Read the model definition and answer for the solid it produces. Units are mm, in the model's axes. A direction names the side the tool comes from. Give positions to 0.01 mm unless a question says otherwise; leave off trailing zeros. Loops run counter-clockwise (first coordinate to the right, second up) from the corner with the lowest first, then second, coordinate; pieces in that order, holes last. Notation, with made-up numbers: (81, -33.75) -> (92, -33.75) arc R20 cw to (92, -10.75) -> close; hole circle Ø4 at (17, 36). An arc over 180 degrees is marked (long way). Return JSON: item names as keys, results as strings. Group by question number.
Autodesk Inventor part; units mm, degrees
ref_plane "YZ Plane" through (0, 0, 0) normal (1, 0, 0) x (0, 1, 0)
ref_plane "XZ Plane" through (0, 0, 0) normal (0, 1, 0) x (-1, 0, 0)
ref_plane "XY Plane" through (0, 0, 0) normal (0, 0, 1) x (1, 0, 0)
sketch "草图2" plane through (0, 0, 0) normal (1, 0, 0) x (0, 1, 0)
  arc A0 (-53.1995, 32.7287) -> (-53.1995, 62.7287) centre (4.8952, 47.7287) ccw
  line L0 (4.8952, 17.7287) -> (24.8952, 17.7287)
  line L1 (24.8952, 17.7287) -> (24.8952, 77.7287)
  line L2 (24.8952, 77.7287) -> (-15.1048, 77.7287)
  line L3 (-15.1048, 77.7287) -> (-15.1048, 17.7287)
  line L4 (-15.1048, 17.7287) -> (4.8952, 17.7287)
  arc A1 (-53.1995, 62.7287) -> (-53.1995, 32.7287) centre (4.8952, 47.7287) ccw
  point P0 (0, 0)
extrude "拉伸2" add sketch "草图2" along normal blind 4
sketch "草图3" plane through (4, 4.8952, 47.7287) normal (1, 0, 0) x (0, 0, -1)
  line L0 (-9, 58) -> (9, 58)
  line L1 (9, 58) -> (9, 54)
  line L2 (9, 54) -> (-9, 54)
  line L3 (-9, 54) -> (-9, 58)
  line L4 (0, -74) -> (0, 175)
  line L5 (0, 0) -> (111.1859, 0)
  line L6 (-9, -58) -> (9, -58)
  line L7 (9, -58) -> (9, -54)
  line L8 (9, -54) -> (-9, -54)
  line L9 (-9, -54) -> (-9, -58)
  line L10 (54, 9) -> (58, 9)
  line L11 (58, 9) -> (58, -9)
  line L12 (58, -9) -> (54, -9)
  line L13 (54, -9) -> (54, 9)
  line L14 (-54, 9) -> (-58, 9)
  line L15 (-58, 9) -> (-58, -9)
  line L16 (-58, -9) -> (-54, -9)
  line L17 (-54, -9) -> (-54, 9)
  dimension "d21" = 18
  dimension "d22" = 4
  dimension "d23" = 18
  dimension "d24" = 4
  dimension "d25" = 108
  dimension "d26" = 108
extrude "拉伸3" add sketch "草图3" along normal blind 18
sketch "草图4" plane through (4, -4.1048, -10.2713) normal (0, 0, -1) x (-1, 0, 0)
  line L0 (-4.5, 27) -> (-4.5, -16)
  line L1 (0, 69) -> (0, -51)
  line L2 (0, 0) -> (-18, 0)
  line L3 (0, 18) -> (-18, 18)
  line L4 (2.402, 9) -> (-9.4185, 9) construction
  circle A0 centre (-4.5, 14.5) radius 1.5
  circle A1 centre (-4.5, 3.5) radius 1.5
  point P0 (4, 4.1048)
  point P1 (-2.25, 9)
  dimension "d29" = 4.5
  dimension "d30" = 3
  dimension "d31" = 11
extrude "拉伸4" cut sketch "草图4" against normal blind 200 contours A0 L0 | L0 A0 | A1 L0 | L0 A1
sketch "草图6" plane through (4, -53.1048, 38.7287) normal (0, -1, 0) x (1, 0, 0)
  line L0 (4.5, -6) -> (4.5, 26.379)
  line L1 (0, -51) -> (0, 69)
  line L2 (0, 18) -> (18, 18)
  line L3 (-1.6886, 9) -> (9.3114, 9) construction
  circle A0 centre (4.5, 3.5) radius 1.5
  circle A1 centre (4.5, 14.5) radius 1.5
  point P0 (-4, -38.7287)
  point P1 (2.25, 9)
  dimension "d34" = 4.5
  dimension "d35" = 3
  dimension "d36" = 11
extrude "拉伸5" cut sketch "草图6" against normal blind 200
sketch "草图7" plane through (4, 4.8952, 47.7287) normal (1, 0, 0) x (0, 0, -1)
  line L0 (-22.6667, -29) -> (27.3333, -29)
  line L1 (27.3333, -29) -> (27.3333, -25)
  line L2 (27.3333, -25) -> (-22.6667, -25)
  line L3 (-22.6667, -25) -> (-22.6667, -29)
  line L4 (30, -20) -> (-30, -20)
  line L5 (0, -20) -> (0, -25)
  point P0 (47.7287, -4.8952)
  dimension "d39" = 4
  dimension "d40" = 50
  dimension "d41" = 5
extrude "拉伸6" add sketch "草图7" along normal blind 40
sketch "草图8" plane through (4, -24.1048, 20.3953) normal (0, -1, 0) x (1, 0, 0)
  line L0 (40, 0) -> (40, 50)
  line L1 (40, 50) -> (40, 25)
  line L2 (40, 25) -> (35, 25)
  line L3 (35, 25) -> (35, 21)
  line L4 (35, 25) -> (35, 29)
  line L5 (35, 25) -> (23, 25)
  line L6 (23, 25) -> (23, 21)
  line L7 (23, 25) -> (23, 29)
  circle A0 centre (35, 21) radius 1.5
  circle A1 centre (35, 29) radius 1.5
  circle A2 centre (23, 29) radius 1.5
  circle A3 centre (23, 21) radius 1.5
  point P0 (-4, -20.3953)
  dimension "d44" = 5
  dimension "d46" = 4
  dimension "d50" = 3
  dimension "d51" = 3
  dimension "d52" = 3
extrude "拉伸7" cut sketch "草图8" against normal blind 40
1. Which of the six approach directions +Z, -Z, +X, -X, +Y, -Y give full straight-line access (tool end or side, diameter ignored) to faces 4 (the flat face through (13, 58.895, 48)), 5 (the flat face through (22, -51, 48)), 6 (the flat face through (13, 5, -10.271))?
2. Determine the mould class of faces 1 (the flat face through (13, 61, 38.729)), 2 (the cylindrical face through (1.972, 27.33, 103.376)), 3 (the flat face through (13, 5, -6.271)) for opening direction Z: pulls with the +Z half, pulls with the -Z half, needs draft (parallel to the pull), parting line crosses it, or undercut.
3. Flat-ended cylindrical pins translate along their axes: pin 1 Ø3 at (x, z) = (28, 45) entering from +Y; pin 2 Ø1.2 at (x, y) = (14.5, -50.5) entering from -Z; pin 3 Ø3 at (y, z) = (33.5, 13) entering from -X; pin 4 Ø3 at (x, y) = (2, 10.5) entering from +Z. Find the tip coordinate at first contact, or state that the pin passes through.
4. Section C-C on y = 17 is taken. Determine the outline of the cut face in (x, z), then the cut area to 3 significant figures.
5. Section D-D on x = 17 is taken. Determine the outline of the cut face in (y, z).
6. Section A-A on x = 27 is taken. Determine the outline of the cut face in (y, z), then the cut area to 3 significant figures.
7. Section B-B on z = 59 is taken. Determine the outline of the cut face in (x, y).
8. Straight lines are drawn through the part: line 1 (Y direction, x = 8.5, z = -8.1); line 2 (Z direction, x = 39, y = -22.85); line 3 (X direction, y = 44.5, z = 36). For each, find the intervals that lie inside material, in ascending order. Write a range as from..to.
Completed:
{
 "1": {"face 4": "+Z, -Z, +X", "face 5": "+Z, -Z, +X, -Y", "face 6": "-Z, +X, +Y, -Y"},
 "2": {"face 1": "pulls with the -Z half", "face 2": "parting line crosses it", "face 3": "undercut"},
 "3": {"pin 1": "stops at y = -20.1", "pin 2": "stops at z = 38.73", "pin 3": "stops at x = 0", "pin 4": "stops at z = 107.59"},
 "4": {"outline": "(0, -11.04) -> (4, -11.04) -> (4, 17.73) -> (0, 17.73) -> close; (0, 77.73) -> (4, 77.73) -> (4, 106.49) -> (0, 106.49) -> close", "area": "230 mm²"},
 "5": {"outline": "(-53.1, 38.73) -> (-49.1, 38.73) -> (-49.1, 56.73) -> (-53.1, 56.73) -> close; (-24.1, 20.4) -> (-20.1, 20.4) -> (-20.1, 70.4) -> (-24.1, 70.4) -> close; (-4.1, -10.27) -> (13.9, -10.27) -> (13.9, -6.27) -> (-4.1, -6.27) -> close; (-4.1, 101.73) -> (13.9, 101.73) -> (13.9, 105.73) -> (-4.1, 105.73) -> close; (58.9, 38.73) -> (62.9, 38.73) -> (62.9, 56.73) -> (58.9, 56.73) -> close"},
 "6": {"outline": "(-24.1, 20.4) -> (-20.1, 20.4) -> (-20.1, 39.9) -> (-24.1, 39.9) -> close; (-24.1, 42.9) -> (-20.1, 42.9) -> (-20.1, 47.9) -> (-24.1, 47.9) -> close; (-24.1, 50.9) -> (-20.1, 50.9) -> (-20.1, 70.4) -> (-24.1, 70.4) -> close", "area": "176 mm²"},
 "7": {"outline": "(0, -54.04) -> (4, -54.04) -> (4, -24.1) -> (44, -24.1) -> (44, -20.1) -> (4, -20.1) -> (4, -15.1) -> (0, -15.1) -> close; (0, 24.9) -> (4, 24.9) -> (4, 63.83) -> (0, 63.83) -> close"},
 "8": {"line 1": "y = -4.1..-2.1, 0.9..8.9, 11.9..13.9", "line 2": "z = 20.4..39.9, 42.9..47.9, 50.9..70.4", "line 3": "x = 0..4"}
}
